Here's how the part is built. I have some questions about the finished solid (model axes, mm). Face numbers are marked on the shaded views. Round coordinates to 2 decimals unless told otherwise and drop trailing zeros. Order: outer loops, then holes, each group sorted by start corner. A loop starts at its lowest first (then second) coordinate and runs counter-clockwise, first axis right, second up.
```python
from build123d import *

# Parameters (mm, degrees)
BOSS_EXTRUDE1_DEPTH = 264


with BuildPart() as part:
    # Sketch1 → Boss-Extrude1 (new body)
    with BuildSketch(Plane(origin=(0, 0, 0), x_dir=(0, 0, -1), z_dir=(1, 0, 0))):
        with BuildLine():
            Line((-7.783565859, 51.412547107), (-7.783565859, -51.412547107))
            ThreePointArc((-7.783565859, -51.412547107), (-9.038756106, -54.322189596), (-12.016575568, -55.405754649))
            ThreePointArc((-12.016575568, -55.405754649), (-64.283565859, 0), (-12.016575568, 55.405754649))
            ThreePointArc((-12.016575568, 55.405754649), (-9.038756106, 54.322189596), (-7.783565859, 51.412547107))
        make_face()
        with BuildLine():
            Line((-9.783565859, 51.412547107), (-9.783565859, -51.412547107))
            ThreePointArc((-9.783565859, -51.412547107), (-10.411160983, -52.867368352), (-11.900070714, -53.409150878))
            ThreePointArc((-11.900070714, -53.409150878), (-62.283565859, 0), (-11.900070714, 53.409150878))
            ThreePointArc((-11.900070714, 53.409150878), (-10.411160983, 52.867368352), (-9.783565859, 51.412547107))
        make_face(mode=Mode.SUBTRACT)
    extrude(amount=BOSS_EXTRUDE1_DEPTH)


solid = part.part
```
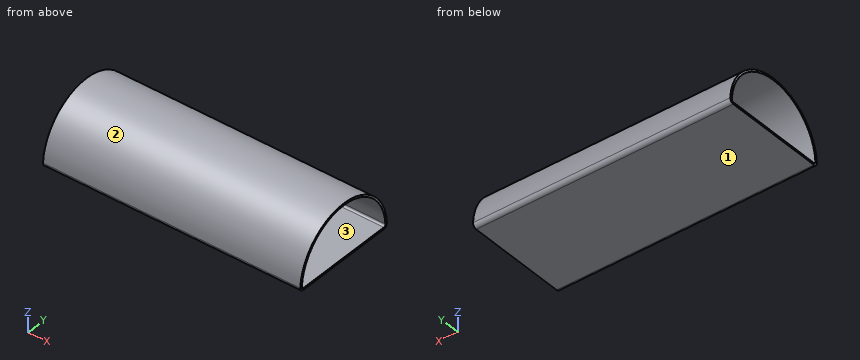
1. If we mould it in two halves opening along Z, with no side actions, what happens to the marked faces 1, 2 and 3? For each: released by +Z, released by -Z, zero draft, split by the parting line, or undercut.
Evaluation:
face 1: released by -Z
face 2: released by +Z
face 3: undercut
2. If we section it at C-C, the plane z = 38: Write out the boundary of the cut face in (x, y), and give its area (3 significant figures).
Evaluation:
outline: (0, -47.19) - (264, -47.19) - (264, -44.82) - (0, -44.82) - close; (0, 44.82) - (264, 44.82) - (264, 47.19) - (0, 47.19) - close
area: 1,250 mm2
3. If we section it at A-A, the plane y = 0: Write out the boundary of the cut face in (x, z), and give its area (3 significant figures).
Evaluation:
outline: (0, 7.78) - (264, 7.78) - (264, 9.78) - (0, 9.78) - close; (0, 62.28) - (264, 62.28) - (264, 64.28) - (0, 64.28) - close
area: 1,060 mm2
4. I'm going to push flat-ended pins straight in: P1, Ø1, axis at x = 205, y = -21, coming from the +Z side; P2, Ø2, axis at x = 232.5, z = 57.5, coming from the +Y side; P3, Ø4, axis at x = 57, y = 2.5, coming from the +Z side; P4, Ø12, axis at y = -28.5, z = 58, coming from the +X side. Where does each tip first touch, or does it pass through?
Evaluation:
P1: stops at z = 60.36
P2: stops at y = 28.34
P3: stops at z = 64.28
P4: stops at x = 264
5. If we section it at B-B, the plane x = 247.5: Write out the boundary of the cut face in (y, z), and give its area (3 significant figures).
Evaluation:
outline: (-55.41, 12.02) arc R4 ccw to (-51.41, 7.78) - (51.41, 7.78) arc R4 ccw to (55.41, 12.02) arc R55.5 ccw to start; hole (-53.41, 11.9) arc R2 ccw to (-51.41, 9.78) - (51.41, 9.78) arc R2 ccw to (53.41, 11.9) arc R53.5 ccw to start
area: 555 mm2
6. I need wall thicknesses on probe 1 along Z at (x, y) = (220, 1); probe 2 along Y at (x, z) = (62, 44.5); probe 3 along Z at (x, y) = (76, 47.5). Which ranges of each line are inside material? Lowest first, please.
Evaluation:
probe 1: z = 7.78 to 9.78, 62.27 to 64.27
probe 2: y = -42.48 to -39.83, 39.83 to 42.48
probe 3: z = 7.78 to 9.78, 33.4 to 37.49
